from build123d import *

# Parameters (mm, degrees)
SKETCH1_R           = 1.389
SKETCH1_R_2         = 0.889
BOSS_EXTRUDE1_DEPTH = 100
SKETCH2_R           = 2.5
BOSS_EXTRUDE2_DEPTH = 50


with BuildPart() as part:
    # Sketch1 → Boss-Extrude1 (new body)
    with BuildSketch(Plane(origin=(0, 0, 0), x_dir=(1, 0, 0), z_dir=(0, 1, 0))):
        Circle(SKETCH1_R)
        Circle(SKETCH1_R_2, mode=Mode.SUBTRACT)
    extrude(amount=BOSS_EXTRUDE1_DEPTH)

    # Sketch2 → Boss-Extrude2 (add)
    with BuildSketch(Plane(origin=(0, 0, 0), x_dir=(1, 0, 0), z_dir=(0, 1, 0))):
        Circle(SKETCH2_R)
    extrude(amount=BOSS_EXTRUDE2_DEPTH)


solid = part.part
The listing builds one solid part. Answer for the finished solid, in the listing's coordinates (mm). A direction names the side the tool comes from. Round coordinates to 2 decimals unless told otherwise and drop trailing zeros. Loops run counter-clockwise (first coordinate to the right, second up) from the corner with the lowest first, then second, coordinate; pieces in that order, holes last. Notation, with made-up numbers: M -7.5,69.25 L 3.5,69.25 A19 ccw 3.5,79.25 Z; hole C 22,65 d5. An arc over 180 degrees is marked long. Return JSON: item names as keys, results as strings.
Q1. Which of the six approach directions +Z, -Z, +X, -X, +Y, -Y give full straight-line access (tool end or side, diameter ignored) to faces 1 (the face through (-0.54, 24.65, 2.44)), 2 (the face through (1.1, 50, 1.1))?
Results list:
{"face 1": "+Y, -Y", "face 2": "+Y"}
Q2. Find section B-B, the plane z = 0. Determine the outline of the cut face in (x, y).
Results list:
{"outline": "M -2.5,0 L 2.5,0 L 2.5,50 L 1.39,50 L 1.39,100 L 0.89,100 L 0.89,50 L -0.89,50 L -0.89,100 L -1.39,100 L -1.39,50 L -2.5,50 Z"}
Q3. Find section C-C, the plane y = 64.5. Determine the outline of the cut face in (x, z).
Results list:
{"outline": "C 0,0 d2.78; hole C 0,0 d1.78"}
Q4. Find section A-A, the plane x = 0. Determine the outline of the cut face in (y, z).
Results list:
{"outline": "M 0,-2.5 L 50,-2.5 L 50,-1.39 L 100,-1.39 L 100,-0.89 L 50,-0.89 L 50,0.89 L 100,0.89 L 100,1.39 L 50,1.39 L 50,2.5 L 0,2.5 Z"}
Q5. Find section D-D, the plane y = 13. Determine the outline of the cut face in (x, z), plus the area to 3 significant figures.
Results list:
{"outline": "C 0,0 d5", "area": "19.6 mm2"}
Q6. Each of these flat-tipped pins is pushed along its axis until it touches: pin 1 Ø1.4 at (x, z) = (0, 0) entering from +Y; pin 2 Ø1 at (x, y) = (-1, 44.5) entering from +Z. Where does it stop, or does it pass through?
Results list:
{"pin 1": "stops at y = 50", "pin 2": "stops at z = 2.45"}
Q7. Find the intervals of material crossed by line 1 along X through (y, z) = (74, 0); line 2 along Y through (x, z) = (-1.6, -0.9), in increasing order. Write a range as from..to.
Results list:
{"line 1": "x = -1.39..-0.89, 0.89..1.39", "line 2": "y = 0..50"}
Q8. The mould has two halves that part along X. Classify faces 3 (the face through (1.325, 74.65, -0.417)), 4 (the face through (0, 50, 0)), 5 (the face through (0, 0, 0)): released by +X, released by -X, zero draft, split by the parting line, or undercut.
Results list:
{"face 3": "split by the parting line", "face 4": "undercut", "face 5": "zero draft"}
